Autodesk Inventor part; units mm, degrees
ref_plane "РабПлоскость1" through (25, 2, 0) normal (1, 0, 0) x (0, 0, -1)
ref_plane "РабПлоскость2" through (2, 12.5, 0) normal (0, -1, 0) x (1, 0, 0)
ref_plane "YZ Plane" through (0, 0, 0) normal (1, 0, 0) x (0, 1, 0)
sketch "Эскиз1" plane through (0, 0, 0) normal (0, 0, 1) x (1, 0, 0)
  line L0 (0, 0) -> (50, 0)
  line L1 (50, 0) -> (50, 25)
  line L2 (50, 25) -> (0, 25)
  line L3 (0, 25) -> (0, 0)
  dimension "d0" = 50
  dimension "d1" = 25
extrude "Выдавливание1" add sketch "Эскиз1" along normal blind 5.2
shell "Оболочка1" thickness 2 removed faces 1 at (16.6667, 16.6667, 0)
sketch "Эскиз2" plane through (0, 0, 5.2) normal (0, 0, 1) x (1, 0, 0)
  line L0 (50, 25) -> (0, 25)
  line L1 (25, 25) -> (25, 0)
  line L2 (0, 0) -> (50, 0)
  line L3 (25, 12.5) -> (12, 12.5)
  line L4 (0, 25) -> (0, 0)
  circle A0 centre (12, 12.5) radius 8.1
  circle A1 centre (38, 12.5) radius 8.1
  line L5 (25, 25) -> (25, 20)
  line L6 (21.75, 20) -> (28.25, 20) construction
  line L7 (21.75, 18) -> (28.25, 18)
  line L8 (28.25, 22) -> (21.75, 22)
  arc A2 (21.75, 22) -> (21.75, 18) centre (21.75, 20) ccw
  arc A3 (28.25, 18) -> (28.25, 22) centre (28.25, 20) ccw
  point P0 (25, 18)
  point P1 (25, 22)
  dimension "d5" = 13
  dimension "d6" = 16.2
  dimension "d9" = 5
  dimension "d10" = 3.25
  dimension "d11" = 4
extrude "Выдавливание2" cut sketch "Эскиз2" against normal through all contours L8 A3 L7 L1 | L1 L7 A2 L8 | A0 | A1
sketch "Эскиз5" plane through (48, 23, 3.2) normal (0, 0, -1) x (-1, 0, 0)
  line L0 (0, 0) -> (1.05, 0)
  line L1 (0, 0) -> (46, 0)
  line L2 (1.05, 0) -> (1.05, -1.05)
  circle A0 centre (1.05, -1.05) radius 1.05
  line L3 (2.1, -2.1) -> (0, -2.1)
  line L4 (0, -2.1) -> (0, 0)
  line L5 (0, 0) -> (2.1, 0)
  line L6 (2.1, 0) -> (2.1, -2.1)
  line L7 (2.1, -2.1) -> (0, 0) construction
  line L8 (0, -2.1) -> (2.1, 0) construction
  point P0 (48, -23)
  point P1 (1.05, -2.1)
  point P2 (2.1, -1.05)
  dimension "d17" = 1.05
  dimension "d18" = 1.05
extrude "Выдавливание4" add sketch "Эскиз5" along normal blind 1 contours L0 A0 L4 | L1 L6 A0 | A0 | A0 L3 L4
ref_plane "РабПлоскость1" through (25, 2, 0) normal (1, 0, 0) x (0, 0, -1)
ref_plane "РабПлоскость2" through (2, 12.5, 0) normal (0, -1, 0) x (1, 0, 0)
mirror "Зеркальное отражение1" about plane through (2, 12.5, 0) normal (0, -1, 0) of "Выдавливание4"
mirror "Зеркальное отражение2" about plane through (25, 2, 0) normal (1, 0, 0) of "Выдавливание4", "Зеркальное отражение1"
sketch "Эскиз14" plane through (0, 0, 0) normal (0, -1, 0) x (1, 0, 0)
  line L0 (35.6735, 8.06) -> (14.3265, 2.34)
  line L1 (14.3265, 2.34) -> (17.8206, -10.6999)
  line L2 (17.8206, -10.6999) -> (39.1675, -4.98)
  line L3 (39.1675, -4.98) -> (35.6735, 8.06)
  line L4 (35.6735, 8.06) -> (17.8206, -10.6999) construction
  line L5 (14.3265, 2.34) -> (39.1675, -4.98) construction
  line L6 (0, 5.2) -> (50, 5.2)
  point P0 (0, 0)
  point P1 (26.747, -1.32)
  point P2 (25, 5.2)
  dimension "d67" = 13.5
  dimension "d68" = 22.1
  dimension "d77" = 15
extrude "Выдавливание10" add sketch "Эскиз14" along normal blind 8
sketch "Эскиз15" plane through (0, -8, 0) normal (0, -1, 0) x (1, 0, 0)
  line L0 (17.8206, -10.6999) -> (39.1675, -4.98)
  line L1 (19.2348, -8.2505) -> (36.718, -3.5658)
  line L2 (36.718, -3.5658) -> (34.2593, 5.6105)
  line L3 (34.2593, 5.6105) -> (16.776, 0.9258)
  line L4 (16.776, 0.9258) -> (19.2348, -8.2505)
  line L5 (39.1675, -4.98) -> (35.6735, 8.06)
  line L6 (17.8206, -10.6999) -> (39.1675, -4.98)
  line L7 (35.6735, 8.06) -> (14.3265, 2.34)
  line L8 (39.1675, -4.98) -> (14.3265, 2.34) construction
  line L9 (17.8206, -10.6999) -> (35.6735, 8.06) construction
  line L10 (19.2348, -8.2505) -> (34.2593, 5.6105) construction
  line L11 (16.776, 0.9258) -> (36.718, -3.5658) construction
  line L12 (34.2593, 5.6105) -> (33.7416, 7.5423)
  line L13 (16.776, 0.9258) -> (16.2584, 2.8577)
  point P0 (0, 0)
  point P1 (26.747, -1.32)
  dimension "d78" = 2
  dimension "d79" = 2
extrude "Выдавливание11" cut sketch "Эскиз15" against normal blind 6
sketch "Эскиз16" plane through (37.8331, 0, 0) normal (0.9659258, 0, 0.258819) x (0.258819, 0, -0.9659258)
  line L0 (5.1557, 0) -> (0, 0)
  line L1 (-5.3834, 0) -> (0, 0)
  line L2 (-8.3443, 0) -> (-8.3443, -8)
  line L3 (5.1557, -8) -> (-8.3443, -8)
  line L4 (5.1557, 0) -> (5.1557, -8)
  line L5 (-5.3834, 0) -> (-8.3443, 0)
  point P0 (-9.7919, 0)
extrude "Выдавливание12" add sketch "Эскиз16" along normal blind 1.5
sketch "Эскиз17" plane through (17.8206, -8, -10.6999) normal (-0.9659258, 0, -0.258819) x (-0.258819, 0, 0.9659258)
  line L0 (2, 0) -> (13.5, 0)
  line L1 (2, 0) -> (2, 6)
  line L2 (2, 6) -> (13.5, 6)
  line L3 (13.5, 0) -> (13.5, 6)
  line L4 (7.75, 6) -> (7.75, 0)
  line L5 (13.5, 0) -> (0, 0)
  point P0 (14.9477, 8)
  point P1 (7.75, 3)
hole "Отверстие4" at (15.8147, -5, -3.214) direction (0.9659258, 0, 0.258819) diameter 2 depth 2
sketch "Эскиз18" plane through (0, 0, 0) normal (0, 1, 0) x (1, 0, 0)
  line L0 (25, -5.2) -> (37.9927, -5.2)
  line L1 (25, -5.2) -> (37.1224, -8.4482)
  line L2 (37.9927, -5.2) -> (37.1224, -8.4482)
  point P0 (0, 0)
extrude "Выдавливание13" cut sketch "Эскиз18" against normal through all
sketch "Эскиз19" plane through (0, 0, 0) normal (0, -1, 0) x (1, 0, 0)
  line L0 (14.3265, 2.34) -> (25, 5.2)
  line L1 (14.3265, 2.34) -> (13.5602, 5.2)
  line L2 (0, 5.2) -> (25, 5.2)
  line L3 (14.3265, 2.34) -> (17.8206, -10.6999)
  line L4 (16.2584, 2.8577) -> (14.3265, 2.34)
  line L5 (16.2584, 2.8577) -> (15.6308, 5.2)
  line L6 (50, 5.2) -> (0, 5.2)
  line L7 (19.2348, -8.2505) -> (16.2584, 2.8577)
  point P0 (0, 0)
extrude "Выдавливание14" add sketch "Эскиз19" along normal up to surface (8 mm away) contours L1 L2 L5 L0
sketch "Эскиз21" plane through (15.6308, 0, 5.2) normal (0, -1, 0) x (1, 0, 0)
  line L0 (0, 0) -> (0.6276, -2.3423)
  line L1 (0.6276, -2.3423) -> (9.3692, 0)
  line L2 (0, 0) -> (9.3692, 0)
  point P0 (-15.6308, -5.2)
extrude "Выдавливание15" add sketch "Эскиз21" along normal up to surface (2 mm away)
properties part number "Крепление ультрасоника вертикальная"
Model file for the job. Use its own axes, mm. A direction names the side the tool comes from. Round coordinates to 2 decimals unless told otherwise and drop trailing zeros. Loops run counter-clockwise (first coordinate to the right, second up) from the corner with the lowest first, then second, coordinate; pieces in that order, holes last. Notation, with made-up numbers: M -30,-23 L -8,-23 A8 cw -8,-15 Z; hole C -13,-7.75 d3. An arc over 180 degrees is marked long. Put each result on its own line as item: value. Start each with the question number.
Item 1: Cut at B-B (x = 12). List the corners of the cut face in (y, z).
Item 2: Mould opens along Y. For faces 4 (the face through (44, 0, 3)), 5 (the face through (25, 25, 3)), 6 (the face through (39.286, -3.944, 0.373)), 7 (the face through (2, 13, 2)) say: released by +Y, released by -Y, zero draft, split by the parting line, or undercut.
Item 3: 3-axis set-ups, long thin cutter, end or side, ignore diameter. For faces 1 (the face through (29, -8, -6)), 2 (the face through (19.75, 20.04, 4.21)), 3 (the face through (45.9, 2.5, 2.7)): which of +Z, -Z, +X, -X, +Y, -Y reach the whole face in a straight line?
Item 4: Cut at C-C (y = 20). List the corners of the cut face in (x, z).
Item 5: Cut at A-A (y = 12.5). List the corners of the cut face in (x, z), then the cut area to 3 significant figures.
Item 6: Cut at D-D (y = -0.5). List the corners of the cut face in (x, z), then the cut area to 3 significant figures.
Item 7: Drop flat-ended pins along their axis: P1, Ø1.6, axis at x = 10, z = 4, coming from the -Y side; P2, Ø1.1, axis at y = 2.5, z = 2.5, coming from the -X side; P3, Ø2.5, axis at x = 28.5, z = 1.5, coming from the -Y side; P4, Ø12.5, axis at x = 25.5, y = 9, coming from the -Z side. Give the stop position or say it passes through.
Item 8: Drill centre lines: line 1 along Y through (x, z) = (38, 4.75); line 2 along Y through (x, z) = (12, 4.1); line 3 along Z through (x, y) = (21, 1). Where is each one in solid material? Low to high.
Answer block:
1. outline: M 0,0 L 2,0 L 2,3.2 L 4.4,3.2 L 4.4,5.2 L 0,5.2 Z; M 20.6,3.2 L 23,3.2 L 23,0 L 25,0 L 25,5.2 L 20.6,5.2 Z
2. face 4: released by -Y
2. face 5: released by +Y
2. face 6: zero draft
2. face 7: undercut
3. face 1: +Z, -Z, +X, -X, -Y
3. face 2: +Z, -Z
3. face 3: -Z
4. outline: M 0,0 L 2,0 L 2,3.2 L 8.94,3.2 L 8.94,5.2 L 0,5.2 Z; M 15.06,3.2 L 19.75,3.2 L 19.75,5.2 L 15.06,5.2 Z; M 30.25,3.2 L 34.94,3.2 L 34.94,5.2 L 30.25,5.2 Z; M 41.06,3.2 L 48,3.2 L 48,0 L 50,0 L 50,5.2 L 41.06,5.2 Z
5. outline: M 0,0 L 2,0 L 2,3.2 L 3.9,3.2 L 3.9,5.2 L 0,5.2 Z; M 20.1,3.2 L 29.9,3.2 L 29.9,5.2 L 20.1,5.2 Z; M 46.1,3.2 L 48,3.2 L 48,0 L 50,0 L 50,5.2 L 46.1,5.2 Z
5. area: 48.0 mm2
6. outline: M 13.56,5.2 L 14.33,2.34 L 17.82,-10.7 L 39.17,-4.98 L 40.62,-4.59 L 37.99,5.2 Z
6. area: 314 mm2
7. P1: y = 0
7. P2: x = 0
7. P3: y = -2
7. P4: z = 3.2
8. line 1: -8 to 4.4, 20.6 to 25
8. line 2: 0 to 4.4, 20.6 to 25
8. line 3: 0 to 5.2
